Autodesk Inventor part; units mm, degrees
ref_plane "YZ Plane" through (0, 0, 0) normal (1, 0, 0) x (0, 1, 0)
ref_plane "XZ Plane" through (0, 0, 0) normal (0, 1, 0) x (-1, 0, 0)
ref_plane "XY Plane" through (0, 0, 0) normal (0, 0, 1) x (1, 0, 0)
sketch "Sketch2" plane through (0, 0, 0) normal (0, 1, 0) x (-1, 0, 0)
  circle A0 centre (0, 0) radius 80 construction
  line L0 (77.2741, 20.7055) -> (103.156, -75.8871)
  line L1 (-77.2741, -20.7055) -> (-51.3922, -117.2981)
  line L2 (103.156, -75.8871) -> (-51.3922, -117.2981) construction
  line L3 (103.156, -75.8871) -> (103.156, -235.8871) construction
  line L4 (103.156, -235.8871) -> (-51.3922, -194.476) construction
  line L5 (-51.3922, -117.2981) -> (-51.3922, -194.476)
  circle A1 centre (0, -311.7741) radius 80 construction
  line L6 (-51.3922, -194.476) -> (-77.2741, -291.0686)
  line L7 (103.156, -235.8871) -> (77.2741, -332.4796)
  arc A2 (77.2741, 20.7055) -> (-77.2741, -20.7055) centre (0, 0) ccw
  arc A3 (-77.2741, -291.0686) -> (77.2741, -332.4796) centre (0, -311.7741) ccw
  circle A4 centre (0, 0) radius 7
  circle A5 centre (0, -311.7741) radius 7
  line L8 (83.156, -48.3871) -> (-31.844, -48.3871)
  line L9 (-31.844, -48.3871) -> (-31.844, -263.3871)
  line L10 (-31.844, -263.3871) -> (83.156, -263.3871)
  line L11 (83.156, -263.3871) -> (83.156, -48.3871)
  arc A6 (103.156, -235.8871) -> (103.156, -75.8871) centre (-201.516, -155.8871) ccw
  circle A7 centre (98.32, -155.8871) radius 7
  point P0 (103.156, -155.8871)
  point P1 (83.156, -155.8871)
  dimension "d0" = 160
  dimension "d1" = 100
  dimension "d2" = 100
  dimension "d3" = 160
  dimension "d4" = 160
  dimension "d5" = 160
  dimension "d6" = 75
  dimension "d7" = 75
  dimension "d8" = 160
  dimension "d9" = 100
  dimension "d10" = 100
  dimension "d11" = 14
  dimension "d12" = 14
  dimension "d13" = 115
  dimension "d14" = 215
  dimension "d15" = 20
  dimension "d39" = 315
  dimension "d40" = 14
  dimension "d41" = 15.164
extrude "Extrusion1" add sketch "Sketch2" along normal blind 339
sketch "Sketch5" plane through (0, 0, 0) normal (0, -1, 0) x (1, 0, 0)
  circle A0 centre (-98.32, -155.8871) radius 7
  circle A1 centre (0, -311.7741) radius 7
  circle A2 centre (0, 0) radius 7
extrude "Extrusion4" add sketch "Sketch5" against normal blind 5
properties part number "TA001" material "ABS Plastic"
Read the model definition and answer for the solid it produces. Units are mm, in the model's axes. A direction names the side the tool comes from. Give positions to 0.01 mm unless a question says otherwise; leave off trailing zeros. Write each loop counter-clockwise with the first axis right and the second up, starting at its lowest first coordinate (ties: lowest second). Pieces come first, ordered by that corner, then holes. Notation, with made-up numbers: (-30.5, 37) -> (24.5, 37) arc R11 cw to (24.5, 47) -> close; hole circle Ø8 at (-7.5, 69). An arc over 180 degrees is marked (long way). Answer in a Markdown table with one row per item.
1) A tool of negligible diameter and unlimited length cuts with its end or side. For faces 1 (the flat face through (-98, 5, -156)), 2 (the flat face through (49, 339, -153)), 3 (the flat face through (51.392, 167, -155)), 4 (the flat face through (31.844, 167, -154)), from which of +Z, -Z, +X, -X, +Y, -Y can it reach the whole face along a straight path? Write none if from no direction.
Results list:
| item | result |
|---|---|
| face 1 | +Y |
| face 2 | +Z, -Z, +X, -X, +Y |
| face 3 | +X, +Y, -Y |
| face 4 | +Y, -Y |
2) Determine the mould class of faces 5 (the flat face through (49, 0, -153)), 6 (the flat face through (-90.4, 167.1, -283.5)), 7 (the cylindrical face through (-113.48, 167.13, -154.75)), 8 (the flat face through (0, 5, 0)) for opening direction Z: released by +Z, released by -Z, zero draft, split by the parting line, or undercut.
Results list:
| item | result |
|---|---|
| face 5 | zero draft |
| face 6 | released by -Z |
| face 7 | split by the parting line |
| face 8 | undercut |
3) Section D-D on x = -48.5 is taken. Give the vertices of the cut face in (y, z).
Results list:
| item | result |
|---|---|
| outline | (0, -375.4) -> (339, -375.4) -> (339, -263.39) -> (0, -263.39) -> close; (0, -48.39) -> (339, -48.39) -> (339, 63.62) -> (0, 63.62) -> close |
4) Section A-A on x = 0 is taken. Give the vertices of the cut face in (y, z).
Results list:
| item | result |
|---|---|
| outline | (0, -391.77) -> (339, -391.77) -> (339, -318.77) -> (5, -318.77) -> (5, -304.77) -> (339, -304.77) -> (339, -263.39) -> (0, -263.39) -> close; (0, -48.39) -> (339, -48.39) -> (339, -7) -> (5, -7) -> (5, 7) -> (339, 7) -> (339, 80) -> (0, 80) -> close |
5) Straight lines are drawn through the part: line 1 (Z direction, x = 0, y = 192.5); line 2 (X direction, y = 130.5, z = -236.5); line 3 (Z direction, x = 6, y = 62.5). For each, find the intervals that lie inside material, in ascending order. Write a range as [from, to].
Results list:
| item | result |
|---|---|
| line 1 | [-391.77, -318.77], [-304.77, -263.39], [-48.39, -7], [7, 80] |
| line 2 | [-102.99, -83.16], [31.84, 62.65] |
| line 3 | [-391.55, -315.38], [-308.17, -263.39], [-48.39, -3.61], [3.61, 79.77] |
6) Section C-C on z = 0 is taken. Give the vertices of the cut face in (x, y).
Results list:
| item | result |
|---|---|
| outline | (-82.82, 0) -> (80, 0) -> (80, 339) -> (7, 339) -> (7, 5) -> (-7, 5) -> (-7, 339) -> (-82.82, 339) -> close |
7) Each of these flat-tipped pins is pushed along its axis until it touches: pin 1 Ø3 at (x, z) = (43.5, -49.5) entering from -Y; pin 2 Ø12.5 at (x, z) = (-98.32, -155.89) entering from +Y; pin 3 Ø3 at (x, y) = (-7, 252) entering from -Z; pin 4 Ø1 at (x, y) = (-73, 155) entering from +Z. Where does it stop, or does it pass through?
Results list:
| item | result |
|---|---|
| pin 1 | y = 0 |
| pin 2 | y = 5 |
| pin 3 | z = -391.58 |
| pin 4 | z = 33.82 |
